The listing builds one solid part. Answer for the finished solid, in the listing's coordinates (mm). A direction names the side the tool comes from. Round coordinates to 2 decimals unless told otherwise and drop trailing zeros. Order: outer loops, then holes, each group sorted by start corner. A loop starts at its lowest first (then second) coordinate and runs counter-clockwise, first axis right, second up. Notation, with made-up numbers: M 56.5,27 L 64.5,27 A25 cw 64.5,63 Z; hole C 23,-11 d6. An arc over 180 degrees is marked long. Put each result on its own line as item: value. Start each with the question number.
1. The mould has two halves that part along Z. Classify faces 1 (the face through (1.26, -38.395, 74.93)), 2 (the face through (1, -48, 90)), 3 (the face through (75, -68, 1)), 4 (the face through (1, -46, 1)): +Z half, -Z half, draft (parallel to the pull), parting line (faces both ways), or undercut.
2. Each of these flat-tipped pins is pushed along its axis until it touches: pin 1 Ø1 at (x, z) = (1.5, 57) entering from -Y; pin 2 Ø13.5 at (y, z) = (-68, 16.5) entering from +X; pin 3 Ø1.5 at (x, y) = (6.5, -61.5) entering from -Z; pin 4 Ø1.8 at (y, z) = (-60, 14.5) entering from +X. Where does it stop, or does it pass through?
3. Which of the six approach directions +Z, -Z, +X, -X, +Y, -Y give full straight-line access (tool end or side, diameter ignored) to faces 5 (the face through (-51.3, -68.4, 1.3)), 6 (the face through (1.26, -38.605, -75.07)), 7 (the face through (-75, -68, 1)), 8 (the face through (-90, -39, -82))?
4. The part is cut by section B-B (x = 70.5). Give the vertices of the cut face in (y, z), then the cut area to 3 significant figures.
5. Consider line 1 (X direction, y = -61, z = 15); line 2 (Y direction, x = 57.5, z = 3.5); line 3 (Y direction, x = -32, z = -67). Determine where each line is inside the solid, lowest interval first.
6. The part is cut by section A-A (y = -65.5). Give the vertices of the cut face in (x, z).
7. The part is cut by section C-C (z = -25.5). Give the vertices of the cut face in (x, y).
8. The part is cut by section D-D (y = -42.5). Give the vertices of the cut face in (x, z).
from build123d import *

# Parameters (mm, degrees)
BOSS_EXTRUDE1_DEPTH = 90
CUT_EXTRUDE1_DEPTH  = 180


with BuildPart() as part:
    # Sketch1 → Boss-Extrude1 (new body, symmetric)
    with BuildSketch(Plane.XY):
        Polygon((-55, -61), (-47.5, -76), (-75, -76), (-75, -59.373791994), (-90, -46), (-90, -31), (90, -31), (90, -46), (75, -59.373791994), (75, -76), (47.5, -76), (55, -61), (55, -59.373791994), (-55, -59.373791994), align=None)
    extrude(amount=BOSS_EXTRUDE1_DEPTH, both=True)

    # Sketch2 → Cut-Extrude1 (cut)
    with BuildSketch(Plane(origin=(90, 0, 0), x_dir=(0, 0, -1), z_dir=(1, 0, 0))):
        Polygon((-70, -31), (-80, -46), (80, -46), (70, -31), align=None)
    extrude(amount=-CUT_EXTRUDE1_DEPTH, mode=Mode.SUBTRACT)


solid = part.part
Resolved:
1. face 1: undercut
1. face 2: +Z half
1. face 3: draft
1. face 4: undercut
2. pin 1: y = -59.37
2. pin 2: x = 75
2. pin 3: through
2. pin 4: x = 75.31
3. face 5: +Z, -Z
3. face 6: +X, -X
3. face 7: +Z, -Z, -X, -Y
3. face 8: +Z, -Z, -X, +Y, -Y
4. outline: M -76,-90 L -31,-90 L -31,-70 L -46,-80 L -46,80 L -31,70 L -31,90 L -76,90 Z
4. area: 5,850 mm2
5. line 1: -75 to -55, 55 to 75
5. line 2: -76 to -46
5. line 3: -59.37 to -46
6. outline: M -75,-90 L -52.75,-90 L -52.75,90 L -75,90 Z; M 52.75,-90 L 75,-90 L 75,90 L 52.75,90 Z
7. outline: M -90,-46 L -75,-59.37 L -75,-76 L -47.5,-76 L -55,-61 L -55,-59.37 L 55,-59.37 L 55,-61 L 47.5,-76 L 75,-76 L 75,-59.37 L 90,-46 Z
8. outline: M -90,-90 L 90,-90 L 90,-77.67 L -90,-77.67 Z; M -90,77.67 L 90,77.67 L 90,90 L -90,90 Z
